The model under review builds one solid part; all positions refer to its coordinate system, in mm. A direction names the side the tool comes from. Round coordinates to 2 decimals unless told otherwise and drop trailing zeros. Order: outer loops, then holes, each group sorted by start corner. A loop starts at its lowest first (then second) coordinate and runs counter-clockwise, first axis right, second up. Notation, with made-up numbers: (35.25, 3) -> (74.25, 3) arc R17 cw to (74.25, 20) -> close; hole circle Ø3 at (-36, -18). An arc over 180 degrees is marked (long way). Put each result on its own line as item: value. Start each with the question number.
from build123d import *

# Parameters (mm, degrees)
SKETCH1_W           = 125
SKETCH1_H           = 100
BOSS_EXTRUDE1_DEPTH = 3
SKETCH2_W           = 2
SKETCH2_H           = 100
BOSS_EXTRUDE2_DEPTH = 17
SKETCH3_R           = 3
BOSS_EXTRUDE4_DEPTH = 4
SKETCH4_W           = 13
SKETCH4_H           = 15
CUT_EXTRUDE1_DEPTH  = 2
SKETCH5_W           = 23
SKETCH5_H           = 15
CUT_EXTRUDE2_DEPTH  = 2
SKETCH6_R           = 1.125
CUT_EXTRUDE3_DEPTH  = 22
FILLET1_R           = 5
FILLET2_R           = 5
SKETCH7_W           = 97.170339499
SKETCH7_H           = 76
CUT_EXTRUDE4_DEPTH  = 22
FILLET3_R           = 2.5


with BuildPart() as part:
    # Sketch1 → Boss-Extrude1 (new body)
    with BuildSketch(Plane(origin=(0, 0, 0), x_dir=(1, 0, 0), z_dir=(0, 1, 0))):
        with Locations((14.321748602, -19.715443405)):
            Rectangle(SKETCH1_W, SKETCH1_H)
    extrude(amount=BOSS_EXTRUDE1_DEPTH)

    # Sketch2 → Boss-Extrude2 (add)
    with BuildSketch(Plane(origin=(0, 3, 0), x_dir=(1, 0, 0), z_dir=(0, 1, 0))):
        with Locations((75.821748602, -19.715443405)):
            Rectangle(SKETCH2_W, SKETCH2_H)
        with Locations((-47.178251398, -19.715443405)):
            Rectangle(SKETCH2_W, SKETCH2_H)
    extrude(amount=BOSS_EXTRUDE2_DEPTH)

    # Sketch3 → Boss-Extrude4 (add)
    with BuildSketch(Plane(origin=(0, 3, 0), x_dir=(1, 0, 0), z_dir=(0, 1, 0))):
        with Locations((-41.178251398, -64.715443405)):
            Circle(SKETCH3_R)
        with Locations((-41.178251398, 25.284556595)):
            Circle(SKETCH3_R)
        with Locations((68.315618549, 25.284556595)):
            Circle(SKETCH3_R)
        with Locations((68.315618549, -64.715443405)):
            Circle(SKETCH3_R)
    extrude(amount=BOSS_EXTRUDE4_DEPTH)

    # Sketch4 → Cut-Extrude1 (cut)
    with BuildSketch(Plane.ZY.offset(48.178251398)):
        with Locations((6.215443405, 12.5)):
            Rectangle(SKETCH4_W, SKETCH4_H)
    extrude(amount=-CUT_EXTRUDE1_DEPTH, mode=Mode.SUBTRACT)

    # Sketch5 → Cut-Extrude2 (cut)
    with BuildSketch(Plane(origin=(76.821748602, 0, 0), x_dir=(0, 0, -1), z_dir=(1, 0, 0))):
        with Locations((-47.215443405, 12.5)):
            Rectangle(SKETCH5_W, SKETCH5_H)
    extrude(amount=-CUT_EXTRUDE2_DEPTH, mode=Mode.SUBTRACT)

    # Sketch6 → Cut-Extrude3 (cut)
    with BuildSketch(Plane(origin=(0, 7, 0), x_dir=(1, 0, 0), z_dir=(0, 1, 0))):
        with Locations((-41.178251398, -64.715443405)):
            Circle(SKETCH6_R)
        with Locations((-41.178251398, 25.284556595)):
            Circle(SKETCH6_R)
        with Locations((68.315618549, -64.715443405)):
            Circle(SKETCH6_R)
        with Locations((68.315618549, 25.284556595)):
            Circle(SKETCH6_R)
    extrude(amount=-CUT_EXTRUDE3_DEPTH, mode=Mode.SUBTRACT)

    # Fillet1
    fillet1_edges = [part.edges().sort_by_distance(p)[0] for p in [
        (75.821748602, 20, 69.715443405),
        (-47.178251398, 20, 69.715443405),
        (-47.178251398, 20, -30.284556595),
        (75.821748602, 20, -30.284556595),
    ]]
    fillet(fillet1_edges, radius=FILLET1_R)

    # Fillet2
    fillet2_edges = [part.edges().sort_by_distance(p)[0] for p in [
        (-47.178251398, 20, -0.284556595),
        (-47.178251398, 20, 12.715443405),
        (75.821748602, 20, 58.715443405),
        (75.821748602, 20, 35.715443405),
    ]]
    fillet(fillet2_edges, radius=FILLET2_R)

    # Sketch7 → Cut-Extrude4 (cut)
    with BuildSketch(Plane(origin=(0, 3, 0), x_dir=(1, 0, 0), z_dir=(0, 1, 0))):
        with Locations((14.406918352, -19.715443405)):
            Rectangle(SKETCH7_W, SKETCH7_H)
    extrude(amount=-CUT_EXTRUDE4_DEPTH, mode=Mode.SUBTRACT)

    # Fillet3
    fillet3_edges = [part.edges().sort_by_distance(p)[0] for p in [
        (62.992088101, 3, 19.715443405),
        (14.406918351, 3, -18.284556595),
        (-34.178251398, 3, 19.715443405),
        (14.406918351, 3, 57.715443405),
    ]]
    fillet(fillet3_edges, radius=FILLET3_R)


solid = part.part
Q1. Take a section at B-B on z = 10. Give the boundary of the cut face in (x, y), and give its area (3 significant figures).
Q2. Take a section at C-C on y = 12.5. Give the boundary of the cut face in (x, z), and give its area (3 significant figures).
Q3. Clearance check with flat-ended pins moving along their axes: pin 1 Ø6 at (x, y) = (15, 7.5) entering from +Z; pin 2 Ø3.5 at (x, z) = (-41.18, -25.28) entering from +Y; pin 3 Ø3.5 at (x, z) = (68.32, 64.72) entering from -Y; pin 4 Ø1 at (x, z) = (-47.5, 6.5) entering from +Y. State where each tip first meets the part, or that it passes through.
Q4. Draft analysis for pull direction X (two halves, no side actions). For faces 1 (the face through (75.836, 18.496, -28.859)), 2 (the face through (63.744, 2.287, 19.148)), 3 (the face through (-48.178, 10, 20)), state which applies: +X half, -X half, draft (parallel to the pull), parting line (faces both ways), or undercut.
Q5. For faces 4 (the face through (75.808, 18.574, 34.212)), 5 (the face through (-46.178, 11, 20)), 6 (the face through (15.12, 2.29, -19.04)), list the 3-axis set-ups (+Z, -Z, +X, -X, +Y, -Y) from which the entire face can be reached by the end or side of a thin tool; tool diameter is ignored.
Q6. Wall thickness on probe 1 along X at (y, z) = (8.75, 59); probe 2 along X at (y, z) = (10.75, 11); probe 3 along X at (y, z) = (15.25, 48.5): over which ranges is each line inside the solid? List them lowest first. Write a range as [from, to].
Q7. Take a section at D-D on z = -10.5. Give the boundary of the cut face in (x, y), and give its area (3 significant figures).
Q8. Take a section at A-A on x = -7.5. Give the boundary of the cut face in (y, z), and give its area (3 significant figures).
Calculated:
1. outline: (-48.18, 0) -> (-34.18, 0) -> (-34.18, 0.5) arc R2.5 ccw to (-36.68, 3) -> (-46.18, 3) -> (-46.18, 5) -> (-48.18, 5) -> close; (62.99, 0) -> (76.82, 0) -> (76.82, 20) -> (74.82, 20) -> (74.82, 3) -> (65.49, 3) arc R2.5 ccw to (62.99, 0.5) -> close
1. area: 119 mm²
2. outline: (-48.18, -30.28) -> (-46.18, -30.28) -> (-46.18, -0.28) -> (-48.18, -0.28) -> close; (-48.18, 12.72) -> (-46.18, 12.72) -> (-46.18, 69.72) -> (-48.18, 69.72) -> close; (74.82, -30.28) -> (76.82, -30.28) -> (76.82, 35.72) -> (74.82, 35.72) -> close; (74.82, 58.72) -> (76.82, 58.72) -> (76.82, 69.72) -> (74.82, 69.72) -> close
2. area: 328 mm²
3. pin 1: passes through
3. pin 2: stops at y = 7
3. pin 3: stops at y = 0
3. pin 4: stops at y = 5
4. face 1: draft
4. face 2: undercut
4. face 3: -X half
5. face 4: +X, +Y
5. face 5: +Z, -Z, +Y
5. face 6: +Y
6. probe 1: x = [-48.18, -46.18], [74.82, 76.82]
6. probe 2: x = [74.82, 76.82]
6. probe 3: x = [-48.18, -46.18]
7. outline: (-48.18, 0) -> (-34.18, 0) -> (-34.18, 0.5) arc R2.5 ccw to (-36.68, 3) -> (-46.18, 3) -> (-46.18, 20) -> (-48.18, 20) -> close; (62.99, 0) -> (76.82, 0) -> (76.82, 20) -> (74.82, 20) -> (74.82, 3) -> (65.49, 3) arc R2.5 ccw to (62.99, 0.5) -> close
7. area: 149 mm²
8. outline: (0, -30.28) -> (3, -30.28) -> (3, -20.78) arc R2.5 ccw to (0.5, -18.28) -> (0, -18.28) -> close; (0, 57.72) -> (0.5, 57.72) arc R2.5 ccw to (3, 60.22) -> (3, 69.72) -> (0, 69.72) -> close
8. area: 69.3 mm²
